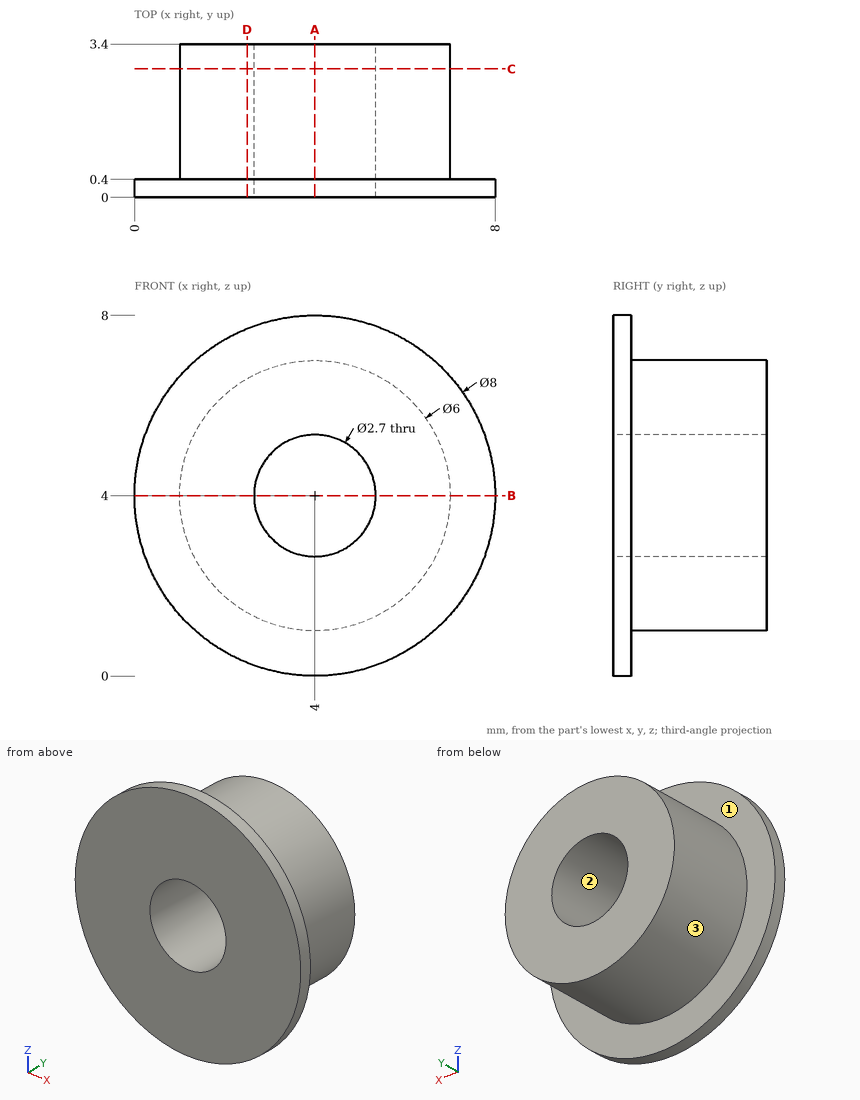
Input: dimensioned drawing with shaded views. Units: mm. Origin: part minimum x, y, z. Give positions to 0.01 mm unless a question says otherwise; leave off trailing zeros. Order: outer loops, then holes, each group sorted by start corner. A loop starts at its lowest first (then second) coordinate and runs counter-clockwise, first axis right, second up. Notation, with made-up numbers: (2, 17.25) -> (38, 17.25) arc R33 cw to (38, 49.25) -> close; hole circle Ø7 at (23.25, -27). An arc over 180 degrees is marked (long way). Write item = value, one per line.
Item 1: Section query D-D (x = 2.5). Output: boundary loops of the cut face in (y, z), then the cut area to 3 significant figures.
Check result:
outline = (0, 0.29) -> (0.4, 0.29) -> (0.4, 1.4) -> (3.4, 1.4) -> (3.4, 6.6) -> (0.4, 6.6) -> (0.4, 7.71) -> (0, 7.71) -> close
area = 18.6 mm²
Item 2: Section query A-A (x = 4). Output: boundary loops of the cut face in (y, z), then the cut area to 3 significant figures.
Check result:
outline = (0, 0) -> (0.4, 0) -> (0.4, 1) -> (3.4, 1) -> (3.4, 2.65) -> (0, 2.65) -> close; (0, 5.35) -> (3.4, 5.35) -> (3.4, 7) -> (0.4, 7) -> (0.4, 8) -> (0, 8) -> close
area = 12.0 mm²
Item 3: Mould query, pull axis Z, two halves, no side actions, for the marked faces 1, 2 and 3. Classes: +Z half, -Z half, draft (parallel to the pull), parting line (faces both ways), or undercut.
Check result:
face_1 = draft
face_2 = undercut
face_3 = parting line
Item 4: Section query C-C (y = 2.85). Output: boundary loops of the cut face in (x, z), then the cut area to 3 significant figures.
Check result:
outline = circle Ø6 at (4, 4); hole circle Ø2.7 at (4, 4)
area = 22.5 mm²
Item 5: Ray query, probe 1 along Z at (x, y) = (4, 1.25); probe 2 along Y at (x, z) = (3, 0.5); probe 3 along X at (y, z) = (0.95, 3.75). Return the intervals inside material, ascending.
Check result:
probe_1 = 1 to 2.65, 5.35 to 7
probe_2 = 0 to 0.4
probe_3 = 1.01 to 2.67, 5.33 to 6.99
Item 6: Section query B-B (z = 4). Output: boundary loops of the cut face in (x, y).
Check result:
outline = (0, 0) -> (2.65, 0) -> (2.65, 3.4) -> (1, 3.4) -> (1, 0.4) -> (0, 0.4) -> close; (5.35, 0) -> (8, 0) -> (8, 0.4) -> (7, 0.4) -> (7, 3.4) -> (5.35, 3.4) -> close
Item 7: Contact query for flat-ended pins moving along their axis: pin 1 (1 mm diameter, centred on y = 1.5, z = 4, fed in from -X); pin 2 (2 mm diameter, centred on x = 7, y = 2, fed in from +Z); pin 3 (4.5 mm diameter, centred on x = 4, z = 4, fed in from -Y); pin 4 (2 mm diameter, centred on x = 3.5, y = 2.5, fed in from -Z). Output: stop coordinate, or through.
Check result:
pin_1 = 1
pin_2 = 6.24
pin_3 = 0
pin_4 = 1
